Input: part model. Units: mm. Frame: model coordinates. A direction names the side the tool comes from. Round coordinates to 2 decimals unless told otherwise and drop trailing zeros. Order: outer loops, then holes, each group sorted by start corner. A loop starts at its lowest first (then second) coordinate and runs counter-clockwise, first axis right, second up. Notation, with made-up numbers: (-17, 3.5) -> (0, 3.5) arc R24 cw to (0, 26.5) -> close; hole circle Ø6 at (55.25, 37). An arc over 180 degrees is marked (long way). Answer as CSV lines item,"result". Start each with the question number.
1) Section query C-C, the plane z = 27.5. Output: boundary loops of the cut face in (x, y).
2) Access query for faces 4 (the face through (53.25, 2, -51)), 5 (the face through (63, 2, 37.5)), 6 (the face through (-63, 2, -45)). Directions: +Z, -Z, +X, -X, +Y, -Y. A direction counts if a zero-diameter tool reaches every point of the face in a straight line with its end or side. Return the directions, or none.
3) Section query B-B, the plane y = 2.7. State how many separate pieces and enclosed holes the cut face has, and give its area (3 significant figures).
4) First-contact query: P1, Ø2.5, axis at x = -32.13, z = 39.96, coming from the +Y side; P2, Ø2.5, axis at x = -61, y = 2, coming from the -Z side; P3, Ø2.5, axis at x = -62, y = 1.5, coming from the +Z side; P4, Ø1.5, axis at y = 2, z = -52, coming from the -X side. Flat tips, straight axial feed; report the tip coordinate or a pass-through.
5) Section query A-A, the plane x = -63.25. Output: boundary loops of the cut face in (y, z), and give its area (4 significant figures).
6) Mould query, pull axis X, two halves, no side actions, for faces 1 (the face through (38.5, 2.5, 2.4)), 2 (the face through (-1, 0, -5)), 3 (the face through (-73.25, 2, -4)). Classes: +X half, -X half, draft (parallel to the pull), parting line (faces both ways), or undercut.
7) Line query: L1, parallel to Z at x = -63.25, y = 2.35; L2, parallel to Z at x = -37.5, y = 2.4; L3, parallel to X at y = 2.7, z = 1.5. Output: solid intervals per line, ascending.
```python
from build123d import *

# Parameters (mm, degrees)
SALIENTE_EXTRUIR1_DEPTH = 5
CROQUIS2_R              = 2.65
CORTAR_EXTRUIR1_DEPTH   = 5
CROQUIS5_R              = 1.5
CROQUIS5_R_2            = 1.445
CORTAR_EXTRUIR2_DEPTH   = 10


with BuildPart() as part:
    # Croquis1 → Saliente-Extruir1 (new body)
    with BuildSketch(Plane(origin=(0, 0, 0), x_dir=(1, 0, 0), z_dir=(0, 1, 0))):
        Polygon((53.25, -50), (53.25, -37.5), (73.25, -37.5), (73.25, 45), (53.25, 45), (53.25, 57.5), (-53.25, 57.5), (-53.25, 45), (-73.25, 45), (-73.25, -37.5), (-53.25, -37.5), (-53.25, -50), align=None)
    extrude(amount=SALIENTE_EXTRUIR1_DEPTH)

    # Croquis2 → Cortar-Extruir1 (cut)
    with BuildSketch(Plane(origin=(0, 5, 0), x_dir=(1, 0, 0), z_dir=(0, 1, 0))):
        with Locations((-63.25, 35)):
            Circle(CROQUIS2_R)
        with Locations((-63.25, -27.5)):
            Circle(CROQUIS2_R)
        with Locations((63.25, 35)):
            Circle(CROQUIS2_R)
        with Locations((63.25, -27.5)):
            Circle(CROQUIS2_R)
    extrude(amount=-CORTAR_EXTRUIR1_DEPTH, mode=Mode.SUBTRACT)

    # Croquis5 → Cortar-Extruir2 (cut)
    with BuildSketch(Plane(origin=(0, 5, 0), x_dir=(1, 0, 0), z_dir=(0, 1, 0))):
        with Locations((-38.797689263, 54.5)):
            Circle(CROQUIS5_R)
        with Locations((39.702310737, 54.5)):
            Circle(CROQUIS5_R)
        with Locations((-38.797689263, -1.5)):
            Circle(CROQUIS5_R)
        with Locations((39.702310737, -1.5)):
            Circle(CROQUIS5_R)
        with Locations((-32.131872623, -39.96)):
            Circle(CROQUIS5_R_2)
        with Locations((-32.131872623, -12)):
            Circle(CROQUIS5_R_2)
        with Locations((20.388127377, -7)):
            Circle(CROQUIS5_R_2)
    extrude(amount=-CORTAR_EXTRUIR2_DEPTH, mode=Mode.SUBTRACT)


solid = part.part
```
Findings:
1,outline,"(-73.25, 0) -> (-65.9, 0) -> (-65.9, 5) -> (-73.25, 5) -> close; (-60.6, 0) -> (60.6, 0) -> (60.6, 5) -> (-60.6, 5) -> close; (65.9, 0) -> (73.25, 0) -> (73.25, 5) -> (65.9, 5) -> close"
2,face 4,"-Z, +X, +Y, -Y"
2,face 5,"+Z, +X, +Y, -Y"
2,face 6,"-Z, -X, +Y, -Y"
3,separate pieces,"1"
3,enclosed holes,"11"
3,area,"14,600 mm^2"
4,P1,"passes through"
4,P2,"stops at z = -45"
4,P3,"stops at z = 37.5"
4,P4,"stops at x = -53.25"
5,outline,"(0, -45) -> (5, -45) -> (5, -37.65) -> (0, -37.65) -> close; (0, -32.35) -> (5, -32.35) -> (5, 24.85) -> (0, 24.85) -> close; (0, 30.15) -> (5, 30.15) -> (5, 37.5) -> (0, 37.5) -> close"
5,area,"359.5 mm^2"
6,face 1,"undercut"
6,face 2,"draft"
6,face 3,"-X half"
7,L1,"z = -45 to -37.65, -32.35 to 24.85, 30.15 to 37.5"
7,L2,"z = -57.5 to -55.25, -53.75 to 0.75, 2.25 to 50"
7,L3,"x = -73.25 to -40.3, -37.3 to 38.2, 41.2 to 73.25"
